Part model, mm, in its own coordinate system. A direction names the side the tool comes from. Round coordinates to 2 decimals unless told otherwise and drop trailing zeros. Write each loop counter-clockwise with the first axis right and the second up, starting at its lowest first coordinate (ties: lowest second). Pieces come first, ordered by that corner, then holes.
1) Saw through at B-B on x = 26.5. Write the cut outline in (y, z).
2) Pull direction Y, two halves, no side cores. Call faces 1 (the flat face through (0, -9.6, 1)), 2 (the flat face through (0, 0, 0)), 3 (the flat face through (0, -6, -8.25)): +Y half, -Y half, draft (parallel to the pull), parting line (faces both ways), or undercut.
3) Saw through at A-A on y = -7.5. Write the cut outline in (x, z), and give its area (3 significant figures).
4) Which spindle directions (+Z, -Z, +X, -X, +Y, -Y) get a long thin tool onto all of the face, cutting with end or side? Do faces 4 (the flat face through (0, -6, -5.75)), 5 (the flat face through (0, -12.1, 0)). Say none if no direction does.
5) Flat gauge pin, fed straight in: pin 1 (6 mm diameter, centred on x = 8.5, y = -9.5, fed in from +Z). Where does the tip first touch, or does it go through?
6) Saw through at C-C on z = 1.25. Write the cut outline in (x, y).
7) Drill centre lines: L1, parallel to Y at x = -4, z = -4.25; L2, parallel to X at y = -9.5, z = 6.5; L3, parallel to Z at x = 23.5, y = -4.5. Where is each one in solid material? Low to high.
```python
from build123d import *

# Parameters (mm, degrees)
F0_W     = 70.3
F0_H     = 16.5
F1_DEPTH = 12.1
F2_T     = -2.5
F3_R     = 1


with BuildPart() as f1:
    # F0 (on Front) → F1 (new body)
    with BuildSketch(Plane.XZ):
        Rectangle(F0_W, F0_H)
    extrude(amount=F1_DEPTH)

    # F2
    f2_openings = [f1.faces().sort_by_distance(p)[0] for p in [
        (0, -6.05, 8.25),
    ]]
    offset(amount=F2_T, openings=f2_openings)

    # F3
    f3_edges = [f1.edges().sort_by_distance(p)[0] for p in [
        (-35.15, -12.1, 0),
        (35.15, -12.1, 0),
        (35.15, 0, 0),
        (-35.15, 0, 0),
    ]]
    fillet(f3_edges, radius=F3_R)


solid = f1.part
```
Completed:
1. outline: (-12.1, -8.25) - (0, -8.25) - (0, 8.25) - (-2.5, 8.25) - (-2.5, -5.75) - (-9.6, -5.75) - (-9.6, 8.25) - (-12.1, 8.25) - close
2. face 1: undercut
2. face 2: +Y half
2. face 3: draft
3. outline: (-35.15, -8.25) - (35.15, -8.25) - (35.15, 8.25) - (32.65, 8.25) - (32.65, -5.75) - (-32.65, -5.75) - (-32.65, 8.25) - (-35.15, 8.25) - close
3. area: 246 mm2
4. face 4: +Z
4. face 5: +Z, -Z, +X, -X, -Y
5. pin 1: stops at z = 8.25
6. outline: (-35.15, -11.1) arc R1 ccw to (-34.15, -12.1) - (34.15, -12.1) arc R1 ccw to (35.15, -11.1) - (35.15, -1) arc R1 ccw to (34.15, 0) - (-34.15, 0) arc R1 ccw to (-35.15, -1) - close; hole (-32.65, -9.6) - (32.65, -9.6) - (32.65, -2.5) - (-32.65, -2.5) - close
7. L1: y = -12.1 to -9.6, -2.5 to 0
7. L2: x = -35.15 to -32.65, 32.65 to 35.15
7. L3: z = -8.25 to -5.75
